The drawing under review shows one solid part. Ordinate dimensions are in mm from its lowest x, y, z. A direction names the side the tool comes from. Give positions to 0.01 mm unless a question says otherwise; leave off trailing zeros. Write each loop counter-clockwise with the first axis right and the second up, starting at its lowest first coordinate (ties: lowest second). Pieces come first, ordered by that corner, then holes.
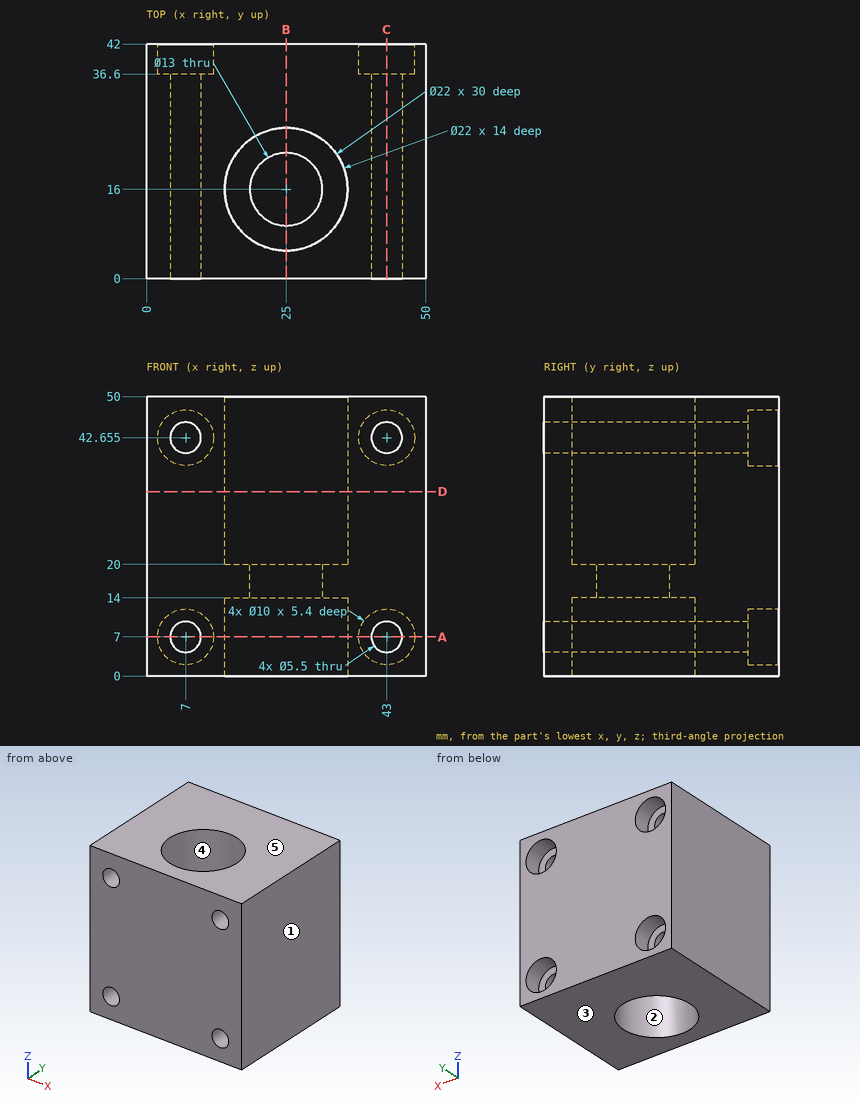
1) To check wall thickness, follow probe 1 along Z at (x, y) = (43, 19) (3 decimals); probe 2 along X at (y, z) = (40.05, 7); probe 3 along Y at (x, z) = (25, 24.5). State the ranges of each line that lie inside material, in increasing order.
2) Consider section D-D, the plane z = 33. Give the boundary of the cut face in (x, y).
3) Consider section B-B, the plane x = 25. Give the boundary of the cut face in (y, z).
4) Consider section C-C, the plane x = 43. Give the boundary of the cut face in (y, z) (3 decimals).
5) Consider section A-A, the plane z = 7. Give the boundary of the cut face in (x, y).
6) Tool access review of the marked faces 4 and 5: name each direction out of +Z, -Z, +X, -X, +Y, -Y from which nothing blocks a thin tool from reaching the whole face with its end or side.
7) The part is to be moulded in two halves that separate along X. For the marked faces 1, 2 and 3, say which applies: +X half, -X half, draft (parallel to the pull), parting line (faces both ways), or undercut.
8) Insertion check: pin 1 (6.5 mm diameter, centred on x = 7, z = 7, fed in from +Y); pin 2 (5 mm diameter, centred on x = 29, y = 10.5, fed in from -Z). Each pin has a flat end and moves straight along its axis. Give the tip position at first contact, or say it passes through.
Answer block:
1. probe 1: z = 0 to 4.25, 9.75 to 39.905, 45.405 to 50
1. probe 2: x = 0 to 2, 12 to 38, 48 to 50
1. probe 3: y = 0 to 5, 27 to 42
2. outline: (0, 0) - (50, 0) - (50, 42) - (0, 42) - close; hole circle Ø22 at (25, 16)
3. outline: (0, 0) - (5, 0) - (5, 14) - (9.5, 14) - (9.5, 20) - (5, 20) - (5, 50) - (0, 50) - close; (22.5, 14) - (27, 14) - (27, 0) - (42, 0) - (42, 50) - (27, 50) - (27, 20) - (22.5, 20) - close
4. outline: (0, 0) - (42, 0) - (42, 2) - (36.6, 2) - (36.6, 4.25) - (0, 4.25) - close; (0, 9.75) - (36.6, 9.75) - (36.6, 12) - (42, 12) - (42, 37.655) - (36.6, 37.655) - (36.6, 39.905) - (0, 39.905) - close; (0, 45.405) - (36.6, 45.405) - (36.6, 47.655) - (42, 47.655) - (42, 50) - (0, 50) - close
5. outline: (0, 0) - (4.25, 0) - (4.25, 36.6) - (2, 36.6) - (2, 42) - (0, 42) - close; (9.75, 0) - (40.25, 0) - (40.25, 36.6) - (38, 36.6) - (38, 42) - (12, 42) - (12, 36.6) - (9.75, 36.6) - close; (45.75, 0) - (50, 0) - (50, 42) - (48, 42) - (48, 36.6) - (45.75, 36.6) - close; hole circle Ø22 at (25, 16)
6. face 4: +Z
6. face 5: +Z, +X, -X, +Y, -Y
7. face 1: +X half
7. face 2: undercut
7. face 3: draft
8. pin 1: stops at y = 36.6
8. pin 2: stops at z = 14
